Input: part model. Units: mm. Frame: model coordinates. A direction names the side the tool comes from. Coordinates: 2 decimals unless noted, no trailing zeros. Loops run counter-clockwise (first coordinate to the right, second up) from the corner with the lowest first, then second, coordinate; pieces in that order, holes last. Notation, with made-up numbers: (-22, -22.75) - (-16, -22.75) arc R8 ccw to (-16, -13.75) - close; hole circle Ø8 at (56.25, -22). An arc over 180 degrees is marked (long way). Answer as CSV lines item,"result". Start each with the question number.
```python
from build123d import *

# Parameters (mm, degrees)
SKETCH1_W           = 16.981866596
SKETCH1_H           = 2.802651254
SKETCH1_R           = 0.825
BOSS_EXTRUDE1_DEPTH = 1
BOSS_EXTRUDE4_DEPTH = 1
BOSS_EXTRUDE5_DEPTH = 1
SKETCH15_W          = 0.931061544
SKETCH15_H          = 1
SKETCH15_W_2        = 0.998936147
BOSS_EXTRUDE6_DEPTH = 9.981867
SKETCH16_W          = 1.5
SKETCH16_H          = 3.5
SKETCH16_W_2        = 1.510044564
BOSS_EXTRUDE7_DEPTH = 1


with BuildPart() as part:
    # Sketch1 → Boss-Extrude1 (new body)
    with BuildSketch(Plane(origin=(0, 0, 0), x_dir=(1, 0, 0), z_dir=(0, 1, 0))):
        with Locations((-27.477281267, 0.001515376)):
            Rectangle(SKETCH1_W, SKETCH1_H)
        with Locations((-34.563340606, 0)):
            Circle(SKETCH1_R, mode=Mode.SUBTRACT)
        with Locations((-20.383340606, 0)):
            Circle(SKETCH1_R, mode=Mode.SUBTRACT)
    extrude(amount=BOSS_EXTRUDE1_DEPTH)

    # Sketch9 → Boss-Extrude4 (add)
    with BuildSketch(Plane(origin=(-23.486347969, 0, 0), x_dir=(0, 0, -1), z_dir=(1, 0, 0))):
        Polygon((1.402841003, 1), (1.402841003, -11.65), (-12.246677238, -11.65), (-12.246677238, -10.65), (-1.399810251, 1), align=None)
        Polygon((-1.399810251, 0), (-11.315615694, -10.65), (-1.399810251, -10.65), align=None, mode=Mode.SUBTRACT)
    extrude(amount=BOSS_EXTRUDE4_DEPTH)

    # Sketch14 → Boss-Extrude5 (add)
    with BuildSketch(Plane.ZY.offset(31.468214565)):
        Polygon((-1.406908915, 1), (-1.406908915, -11.65), (12.242609326, -11.65), (12.242609326, -10.65), (1.395742339, 1), align=None)
        Polygon((11.311547782, -10.65), (1.395742339, -10.65), (1.395742339, 0), align=None, mode=Mode.SUBTRACT)
    extrude(amount=BOSS_EXTRUDE5_DEPTH)

    # Sketch15 → Boss-Extrude6 (add)
    with BuildSketch(Plane(origin=(-22.486347969, 0, 0), x_dir=(0, 0, -1), z_dir=(1, 0, 0))):
        with Locations((-11.781146466, -11.15)):
            Rectangle(SKETCH15_W, SKETCH15_H)
        with Locations((-9.817677681, -11.15)):
            Rectangle(SKETCH15_W_2, SKETCH15_H)
        with Locations((-7.819805388, -11.15)):
            Rectangle(SKETCH15_W_2, SKETCH15_H)
    extrude(amount=-BOSS_EXTRUDE6_DEPTH)

    # Sketch16 → Boss-Extrude7 (add)
    with BuildSketch(Plane.XZ.offset(11.65)):
        with Locations((-24.236347969, 5.570337314)):
            Rectangle(SKETCH16_W, SKETCH16_H)
        with Locations((-30.713192283, 5.570337314)):
            Rectangle(SKETCH16_W_2, SKETCH16_H)
    extrude(amount=-BOSS_EXTRUDE7_DEPTH)


solid = part.part
```
Item 1: Draft query along Y for faces 6 (the flat face through (-27, 1, 0)), 7 (the flat face through (-32, -5, 1.396)), 8 (the flat face through (-27, -11, 8.319)). Return one class per face: pulls with the +Y half, pulls with the -Y half, needs draft (parallel to the pull), parting line crosses it, or undercut.
Item 2: Section query B-B, the plane z = 0. Output: boundary loops of the cut face in (x, y), and give its area (3 significant figures).
Item 3: Set-up query: faces 1 (the flat face through (-31.468, -7, 0)), 2 (the flat face through (-31.961, -5.25, 6.284)), 3 (the flat face through (-20.8, 0.5, 1.4)), 4 (the flat face through (-23.486, -11, 9)), 5 (the flat face through (-24, -11, 3.82)). Return all of +Z, -Z, +X, -X, +Y, -Y with unobstructed straight access to the full face (end or side cutting, diameter ignored); none if empty.
Item 4: Material intervals for probe 1 along X at (y, z) = (0.2, 0); probe 2 along X at (y, z) = (-4.75, 0.25); probe 3 along Y at (x, z) = (-30.25, 5), sorted ascending.
Item 5: Section query C-C, the plane y = -0.75. Output: boundary loops of the cut face in (x, z), and give its area (3 significant figures).
Item 6: Section query D-D, the plane x = -34.5. Output: boundary loops of the cut face in (y, z), and give its area (3 significant figures).
Item 7: Contact query for flat-ended pins moving along their axis: P1, Ø0.5, axis at y = -11, z = 5.5, coming from the +X side; P2, Ø0.8, axis at x = -20.5, z = 0.5, coming from the -Y side; P3, Ø0.5, axis at x = -27, y = -11, coming from the -Z side. Output: stop coordinate, or through.
Item 8: Section query A-A, the plane x = -23.25. Output: boundary loops of the cut face in (y, z).
Response values:
1,face 6,"pulls with the +Y half"
1,face 7,"undercut"
1,face 8,"needs draft"
2,outline,"(-35.97, 0) - (-35.39, 0) - (-35.39, 1) - (-35.97, 1) - close; (-33.74, 0) - (-32.47, 0) - (-32.47, -11.65) - (-31.47, -11.65) - (-31.47, 0) - (-23.49, 0) - (-23.49, -11.65) - (-22.49, -11.65) - (-22.49, 0) - (-21.21, 0) - (-21.21, 1) - (-33.74, 1) - close; (-19.56, 0) - (-18.99, 0) - (-18.99, 1) - (-19.56, 1) - close"
2,area,"37.0 mm²"
3,face 1,"-Z, -Y"
3,face 2,"+X, -X"
3,face 3,"+Z, +X, +Y, -Y"
3,face 4,"+Y, -Y"
3,face 5,"-Z, +Y, -Y"
4,probe 1,"x = -35.97 to -35.39, -33.74 to -21.21, -19.56 to -18.99"
4,probe 2,"x = -32.47 to -31.47, -23.49 to -22.49"
4,probe 3,"y = -11.65 to -10.65"
5,outline,"(-32.47, -1.41) - (-31.47, -1.41) - (-31.47, 1.4) - (-32.47, 1.4) - close; (-32.47, 2.09) - (-31.47, 2.09) - (-31.47, 3.03) - (-32.47, 3.03) - close; (-23.49, -1.4) - (-22.49, -1.4) - (-22.49, 1.4) - (-23.49, 1.4) - close; (-23.49, 2.1) - (-22.49, 2.1) - (-22.49, 3.03) - (-23.49, 3.03) - close"
5,area,"7.47 mm²"
6,outline,"(0, -1.4) - (1, -1.4) - (1, -0.82) - (0, -0.82) - close; (0, 0.82) - (1, 0.82) - (1, 1.4) - (0, 1.4) - close"
6,area,"1.16 mm²"
7,P1,"stops at x = -22.49"
7,P2,"stops at y = 0"
7,P3,"stops at z = 7.32"
8,outline,"(-11.65, -1.4) - (1, -1.4) - (1, 1.4) - (-10.65, 12.25) - (-11.65, 12.25) - close; hole (-10.65, 1.4) - (0, 1.4) - (-10.65, 11.32) - close"
